Autodesk Inventor part; units mm, degrees
ref_plane "YZ Plane" through (0, 0, 0) normal (1, 0, 0) x (0, 1, 0)
ref_plane "XZ Plane" through (0, 0, 0) normal (0, 1, 0) x (-1, 0, 0)
ref_plane "XY Plane" through (0, 0, 0) normal (0, 0, 1) x (1, 0, 0)
sketch "Boceto1" plane through (0, 0, 0) normal (1, 0, 0) x (0, 1, 0)
  line L0 (0, 0) -> (20, 0)
  line L1 (20, 0) -> (20, -1)
  line L2 (20, -1) -> (0, -1)
  line L3 (0, -1) -> (0, 0)
  line L4 (0, 0) -> (1, 0)
  line L5 (1, 0) -> (1, -20)
  line L6 (1, -20) -> (0, -20)
  line L7 (0, -20) -> (0, 0)
  point P0 (1, -1)
  dimension "d0" = 20
  dimension "d1" = 20
  dimension "d2" = 1
  dimension "d3" = 1
extrude "Extrusión1" add sketch "Boceto1" along normal blind 200
sketch "Boceto2" plane through (0, 1, -1) normal (0, 0, -1) x (-1, 0, 0)
  circle A0 centre (-194.35, 15.65) radius 1.75
  line L0 (0, 19) -> (-200, 19)
  line L1 (-200, 0) -> (-200, 19)
  circle A1 centre (-163.35, 15.65) radius 1.75
  point P0 (0, -1)
  dimension "d6" = 3.5
  dimension "d7" = 3.35
  dimension "d8" = 5.65
  dimension "d11" = 3.5
  dimension "d12" = 31
  dimension "d13" = 3.35
extrude "Extrusión2" cut sketch "Boceto2" against normal through all
sketch "Boceto3" plane through (0, 1, -1) normal (0, 1, 0) x (1, 0, 0)
  circle A0 centre (193, 10) radius 1.5
  circle A1 centre (167, 10) radius 1.5
  line L0 (0, 19) -> (200, 19)
  line L1 (200, 19) -> (200, 0)
  point P0 (0, -1)
  dimension "d14" = 3
  dimension "d15" = 3
  dimension "d16" = 9
  dimension "d17" = 9
  dimension "d18" = 7
  dimension "d19" = 26
extrude "Extrusión3" cut sketch "Boceto3" against normal through all
sketch "Boceto4" plane through (0, 0, 0) normal (0, 0, 1) x (1, 0, 0)
  circle A0 centre (65.7, 11) radius 2.5
  line L0 (200, 20) -> (200, 0)
  circle A1 centre (130.7, 11) radius 2.5
  line L1 (0, 20) -> (200, 20)
  point P0 (0, 0)
  dimension "d22" = 134.3
  dimension "d23" = 69.3
  dimension "d24" = 9
  dimension "d25" = 9
  dimension "d28" = 5
  dimension "d29" = 5
extrude "Extrusión4" cut sketch "Boceto4" against normal through all
sketch "Boceto5" plane through (0, 1, -1) normal (0, 1, 0) x (1, 0, 0)
  circle A0 centre (60.7, 10) radius 2.5
  line L0 (0, 19) -> (200, 19)
  line L1 (0, 19) -> (0, 0)
  circle A1 centre (93.2, 10) radius 2.5
  circle A2 centre (141.7, 10) radius 2.5
  point P0 (0, -1)
  dimension "d30" = 5
  dimension "d31" = 9
  dimension "d32" = 60.7
  dimension "d33" = 5
  dimension "d35" = 5
  dimension "d36" = 48.5
  dimension "d39" = 32.5
extrude "Extrusión5" cut sketch "Boceto5" against normal through all
equation "\"d1\" = d0"
equation "\"d3\" = d2"
equation "\"d11\" = d6"
equation "\"d13\" = d7"
equation "\"d15\" = d14"
equation "\"d17\" = d16"
equation "\"d24\" = d25"
equation "\"d29\" = d28"
equation "\"d33\" = d30"
equation "\"d35\" = d33"
properties part number "Angulo 2020x450" material "Madera (cerezo)"
Source: CAD feature listing. Evaluate the final solid. Frame: model axes, mm. A direction names the side the tool comes from. Give positions to 0.01 mm unless a question says otherwise; leave off trailing zeros. Write each loop counter-clockwise with the first axis right and the second up, starting at its lowest first coordinate (ties: lowest second). Pieces come first, ordered by that corner, then holes. Notation, with made-up numbers: (31.5, 9.5) -> (46.5, 9.5) arc R17 cw to (46.5, 27.5) -> close; hole circle Ø10 at (25.25, -21.75). An arc over 180 degrees is marked (long way). Write item = value, one per line.
Q1. Cut plane C-C on z = -18.25. Return loops of the section in (x, y).
Here are the results:
outline = (0, 0) -> (200, 0) -> (200, 1) -> (0, 1) -> close
Q2. Line query: line 1 (Z direction, x = 141.7, y = 0.75); line 2 (Y direction, x = 36.5, z = -9.5); line 3 (Y direction, x = 130.7, z = -0.5). Output: solid intervals per line, ascending. Write a range as from..to.
Here are the results:
line_1 = -20..-13.5, -8.5..0
line_2 = 0..1
line_3 = 0..8.5, 13.5..20
Q3. Cut plane A-A on x = 60.7. Return loops of the section in (y, z).
Here are the results:
outline = (0, -20) -> (1, -20) -> (1, -13.5) -> (0, -13.5) -> close; (0, -8.5) -> (1, -8.5) -> (1, -1) -> (20, -1) -> (20, 0) -> (0, 0) -> close
Q4. Reachability of faces 1 (the face through (99, 1, -10)), 2 (the face through (133.01, 10.04, -0.49)) from +Z, -Z, +X, -X, +Y, -Y: full face, straight path, thin tool, end or side. Return the list, or none.
Here are the results:
face_1 = -Z, +X, -X, +Y
face_2 = +Z, -Z
Q5. Cut plane D-D on x = 16. Return loops of the section in (y, z).
Here are the results:
outline = (0, -20) -> (1, -20) -> (1, -1) -> (20, -1) -> (20, 0) -> (0, 0) -> close
Q6. Mould query, pull axis Z, two halves, no side actions, for faces 3 (the face through (99, 11, -1)), 4 (the face through (195.74, 15.59, -0.51)), 5 (the face through (94.35, 0.51, -8.78)). Classes: +Z half, -Z half, draft (parallel to the pull), parting line (faces both ways), or undercut.
Here are the results:
face_3 = -Z half
face_4 = draft
face_5 = undercut
Q7. Cut plane B-B on x = 163.35. Return loops of the section in (y, z).
Here are the results:
outline = (0, -20) -> (1, -20) -> (1, -1) -> (14.9, -1) -> (14.9, 0) -> (0, 0) -> close; (18.4, -1) -> (20, -1) -> (20, 0) -> (18.4, 0) -> close
Q8. First-contact query: pin 1 (12 mm diameter, centred on x = 151.5, y = 6.5, fed in from -Z); pin 2 (6.5 mm diameter, centred on x = 141.7, z = -11, fed in from +Y); pin 3 (3 mm diameter, centred on x = 115.5, y = 7.5, fed in from -Z). Flat tips, straight axial feed; report the tip coordinate or a pass-through.
Here are the results:
pin_1 = -20
pin_2 = 1
pin_3 = -1
